from build123d import *

# Parameters (mm, degrees)
SKETCH1_R           = 33
BOSS_EXTRUDE1_DEPTH = 1.6
SKETCH2_R           = 1.2
CUT_EXTRUDE1_DEPTH  = 3
SKETCH3_R           = 3.75
CUT_EXTRUDE2_DEPTH  = 3
SKETCH5_R           = 0.39
CUT_EXTRUDE4_DEPTH  = 10
SKETCH6_R           = 3.75
BOSS_EXTRUDE2_DEPTH = 1.7


with BuildPart() as part:
    # Sketch1 → Boss-Extrude1 (new body)
    with BuildSketch(Plane(origin=(0, 0, 0), x_dir=(1, 0, 0), z_dir=(0, 1, 0))):
        with Locations(Location((0, 0, 0), (0, 0, 270))):
            Circle(SKETCH1_R)
    extrude(amount=BOSS_EXTRUDE1_DEPTH)

    # Sketch2 → Cut-Extrude1 (cut)
    with BuildSketch(Plane(origin=(0, 1.6, 0), x_dir=(1, 0, 0), z_dir=(0, 1, 0))):
        with Locations(Location((0, 27.5, 0), (0, 0, 270))):
            Circle(SKETCH2_R)
        with Locations(Location((27.5, 0, 0), (0, 0, 270))):
            Circle(SKETCH2_R)
        with Locations(Location((0, -27.5, 0), (0, 0, 270))):
            Circle(SKETCH2_R)
        with Locations(Location((-27.5, 0, 0), (0, 0, 270))):
            Circle(SKETCH2_R)
    extrude(amount=-CUT_EXTRUDE1_DEPTH, mode=Mode.SUBTRACT)

    # Sketch3 → Cut-Extrude2 (cut)
    with BuildSketch(Plane(origin=(0, 1.6, 0), x_dir=(1, 0, 0), z_dir=(0, 1, 0))):
        with Locations(Location((0, 0, 0), (0, 0, 270))):
            Circle(SKETCH3_R)
    extrude(amount=-CUT_EXTRUDE2_DEPTH, mode=Mode.SUBTRACT)

    # Sketch5 → Cut-Extrude4 (cut)
    with BuildSketch(Plane(origin=(0, 1.6, 0), x_dir=(1, 0, 0), z_dir=(0, 1, 0))):
        with Locations(Location((-1.780167472, 7.799423297, 0), (0, 0, 270))):
            Circle(SKETCH5_R)
        with Locations(Location((1.780167472, 7.799423297, 0), (0, 0, 270))):
            Circle(SKETCH5_R)
        with Locations(Location((4.987918415, 6.25465186, 0), (0, 0, 270))):
            Circle(SKETCH5_R)
        with Locations(Location((7.207750943, 3.471069913, 0), (0, 0, 270))):
            Circle(SKETCH5_R)
        with Locations(Location((8, 0, 0), (0, 0, 270))):
            Circle(SKETCH5_R)
        with Locations(Location((1.780167472, -7.799423297, 0), (0, 0, 270))):
            Circle(SKETCH5_R)
        with Locations(Location((-1.780167472, -7.799423297, 0), (0, 0, 270))):
            Circle(SKETCH5_R)
        with Locations(Location((-4.987918415, -6.25465186, 0), (0, 0, 270))):
            Circle(SKETCH5_R)
        with Locations(Location((-7.207750943, -3.471069913, 0), (0, 0, 270))):
            Circle(SKETCH5_R)
        with Locations(Location((-8, 0, 0), (0, 0, 270))):
            Circle(SKETCH5_R)
        with Locations(Location((-7.207750943, 3.471069913, 0), (0, 0, 270))):
            Circle(SKETCH5_R)
        with Locations(Location((-4.987918415, 6.25465186, 0), (0, 0, 270))):
            Circle(SKETCH5_R)
    extrude(amount=-CUT_EXTRUDE4_DEPTH, mode=Mode.SUBTRACT)

    # Sketch6 → Boss-Extrude2 (add)
    with BuildSketch(Plane(origin=(0, 1.6, 0), x_dir=(1, 0, 0), z_dir=(0, 1, 0))):
        with Locations(Location((0, 0, 0), (0, 0, 270))):
            Circle(SKETCH6_R)
    extrude(amount=-BOSS_EXTRUDE2_DEPTH)


solid = part.part
Geometry check sheet. Reference: the model listing, model coordinates, mm. Give positions to 0.01 mm unless a question says otherwise; leave off trailing zeros. Order: outer loops, then holes, each group sorted by start corner. A loop starts at its lowest first (then second) coordinate and runs counter-clockwise, first axis right, second up. Notation, with made-up numbers: (-27, 68) - (30, 68) arc R17 ccw to (30, 75) - close; hole circle Ø10 at (9, 74). An arc over 180 degrees is marked (long way). Use one line per item in the form item = value.
1) Material ranges on probe 1 along X at (y, z) = (1.05, 0); probe 2 along Z at (x, y) = (2, 1.1); probe 3 along X at (y, z) = (1, 8), recorded low to high. Write a range as from..to.
Working result:
probe_1 = -33..-28.7, -26.3..-8.39, -7.61..7.61, 8.39..26.3, 28.7..33
probe_2 = -32.94..-8.12, -7.48..7.48, 8.12..32.94
probe_3 = -32.02..-2.11, -1.45..1.45, 2.11..32.02
2) Sectioned sample at D-D (x = -27.5). Record the boundary of the cut face in (y, z).
Working result:
outline = (0, -18.24) - (1.6, -18.24) - (1.6, -1.2) - (0, -1.2) - close; (0, 1.2) - (1.6, 1.2) - (1.6, 18.24) - (0, 18.24) - close
3) Sectioned sample at C-C (y = 0.8). Count the separate pieces of the cut face and the enclosed holes in it, and give its area (3 significant figures).
Working result:
separate_pieces = 1
enclosed_holes = 16
area = 3,400 mm^2
4) Sectioned sample at B-B (z = 27.5). Record the boundary of the cut face in (x, y), and give its area (3 significant figures).
Working result:
outline = (-18.24, 0) - (-1.2, 0) - (-1.2, 1.6) - (-18.24, 1.6) - close; (1.2, 0) - (18.24, 0) - (18.24, 1.6) - (1.2, 1.6) - close
area = 54.5 mm^2
5) Sectioned sample at A-A (x = 0). Record the boundary of the cut face in (y, z), and give its area (3 significant figures).
Working result:
outline = (-0.1, -3.75) - (0, -3.75) - (0, -26.3) - (1.6, -26.3) - (1.6, 26.3) - (0, 26.3) - (0, 3.75) - (-0.1, 3.75) - close; (0, -33) - (1.6, -33) - (1.6, -28.7) - (0, -28.7) - close; (0, 28.7) - (1.6, 28.7) - (1.6, 33) - (0, 33) - close
area = 98.7 mm^2
6) Depth check by flat-ended pin: pin 1 Ø2 at (x, z) = (-11.5, -9.5) entering from -Y; pin 2 Ø1.9 at (x, z) = (0, -27.5) entering from +Y; pin 3 Ø1 at (x, y) = (-1, 1) entering from -Z; pin 4 Ø1 at (y, z) = (1, 5.5) entering from -X. Enter the tip coordinate at first touch or a pass-through.
Working result:
pin_1 = 0
pin_2 = through
pin_3 = -33
pin_4 = -32.62
